```python
from build123d import *

# Parameters (mm, degrees)
CROQUIS1_R              = 100
SALIENTE_EXTRUIR1_DEPTH = 3
CROQUIS3_R              = 110
CORTAR_EXTRUIR1_DEPTH   = 3
REDONDEO1_R             = 10
CROQUIS4_R              = 1.5
CORTAR_EXTRUIR2_DEPTH   = 142.453172607
CROQUIS5_R              = 1.25
CROQUIS5_W              = 4.4
CROQUIS5_H              = 7.75
CROQUIS5_W_2            = 7.75
CROQUIS5_H_2            = 4.4
CORTAR_EXTRUIR3_DEPTH   = 142.453172607
CROQUIS6_R              = 20
CORTAR_EXTRUIR4_DEPTH   = 142.453172607


with BuildPart() as part:
    # Croquis1 → Saliente-Extruir1 (new body)
    with BuildSketch(Plane.XY):
        Circle(CROQUIS1_R)
    extrude(amount=SALIENTE_EXTRUIR1_DEPTH)

    # Croquis3 → Cortar-Extruir1 (cut)
    with BuildSketch(Plane.XY.offset(3)):
        with Locations((190, 0)):
            Circle(CROQUIS3_R)
    extrude(amount=-CORTAR_EXTRUIR1_DEPTH, mode=Mode.SUBTRACT)

    # Redondeo1
    redondeo1_edges = [part.edges().sort_by_distance(p)[0] for p in [
        (89.473684211, -44.659375654, 1.5),
        (89.473684211, 44.659375654, 1.5),
    ]]
    fillet(redondeo1_edges, radius=REDONDEO1_R)

    # Croquis4 → Cortar-Extruir2 (cut, through all)
    with BuildSketch(Plane.XY.offset(3)):
        with Locations((-10.995510447, 37.794857454)):
            Circle(CROQUIS4_R)
        with Locations((-51.936993078, -25.137646071)):
            Circle(CROQUIS4_R)
        with Locations((-25.137646071, -51.936993078)):
            Circle(CROQUIS4_R)
        with Locations((-10.995510447, -37.794857454)):
            Circle(CROQUIS4_R)
        with Locations((-37.794857454, -10.995510447)):
            Circle(CROQUIS4_R)
        with Locations((-37.794857454, 10.995510447)):
            Circle(CROQUIS4_R)
        with Locations((-51.936993078, 25.137646071)):
            Circle(CROQUIS4_R)
        with Locations((-25.137646071, 51.936993078)):
            Circle(CROQUIS4_R)
        with Locations((37.794857454, 10.995510447)):
            Circle(CROQUIS4_R)
        with Locations((10.995510447, 37.794857454)):
            Circle(CROQUIS4_R)
        with Locations((25.137646071, 51.936993078)):
            Circle(CROQUIS4_R)
        with Locations((51.936993078, 25.137646071)):
            Circle(CROQUIS4_R)
        with Locations((10.995510447, -37.794857454)):
            Circle(CROQUIS4_R)
        with Locations((37.794857454, -10.995510447)):
            Circle(CROQUIS4_R)
        with Locations((51.936993078, -25.137646071)):
            Circle(CROQUIS4_R)
        with Locations((25.137646071, -51.936993078)):
            Circle(CROQUIS4_R)
        Polygon((-83.085046789, -58.336309448), (-58.336309448, -83.085046789), (-43.487067043, -68.235804385), (-68.235804385, -43.487067043), align=None)
        Polygon((-58.336309448, 83.085046789), (-43.487067043, 68.235804385), (-68.235804385, 43.487067043), (-83.085046789, 58.336309448), align=None)
        Polygon((83.085046789, 58.336309448), (68.235804385, 43.487067043), (43.487067043, 68.235804385), (58.336309448, 83.085046789), align=None)
        Polygon((58.336309448, -83.085046789), (43.487067043, -68.235804385), (68.235804385, -43.487067043), (83.085046789, -58.336309448), align=None)
    extrude(amount=-CORTAR_EXTRUIR2_DEPTH, mode=Mode.SUBTRACT)

    # Croquis5 → Cortar-Extruir3 (cut, through all)
    with BuildSketch(Plane.XY.offset(3)):
        with Locations((-86, 18.59)):
            Circle(CROQUIS5_R)
        with Locations((-77, 18.59)):
            Circle(CROQUIS5_R)
        with Locations(Location((-77, -18.59, 0), (0, 0, 180))):
            Circle(CROQUIS5_R)
        with Locations(Location((-86, -18.59, 0), (0, 0, 180))):
            Circle(CROQUIS5_R)
        with Locations((18.59, 77)):
            Circle(CROQUIS5_R)
        with Locations((18.59, 86)):
            Circle(CROQUIS5_R)
        with Locations(Location((-18.59, 86, 0), (0, 0, 180))):
            Circle(CROQUIS5_R)
        with Locations(Location((-18.59, 77, 0), (0, 0, 180))):
            Circle(CROQUIS5_R)
        with Locations((62, 18.59)):
            Circle(CROQUIS5_R)
        with Locations((71, 18.59)):
            Circle(CROQUIS5_R)
        with Locations((62, -18.59)):
            Circle(CROQUIS5_R)
        with Locations((71, -18.59)):
            Circle(CROQUIS5_R)
        with Locations((-18.59, -77)):
            Circle(CROQUIS5_R)
        with Locations((-18.59, -86)):
            Circle(CROQUIS5_R)
        with Locations(Location((18.59, -86, 0), (0, 0, 180))):
            Circle(CROQUIS5_R)
        with Locations(Location((18.59, -77, 0), (0, 0, 180))):
            Circle(CROQUIS5_R)
        with Locations((-14.64, 82.125)):
            Rectangle(CROQUIS5_W, CROQUIS5_H)
        with Locations((-80.875, 14.64)):
            Rectangle(CROQUIS5_W_2, CROQUIS5_H_2)
        with Locations((67.125, 14.64)):
            Rectangle(CROQUIS5_W_2, CROQUIS5_H_2)
        with Locations((-14.64, -80.875)):
            Rectangle(CROQUIS5_W, CROQUIS5_H)
    extrude(amount=-CORTAR_EXTRUIR3_DEPTH, mode=Mode.SUBTRACT)

    # Croquis6 → Cortar-Extruir4 (cut, through all)
    with BuildSketch(Plane(origin=(0, 0, 0), x_dir=(-1, 0, 0), z_dir=(0, 0, -1))):
        Circle(CROQUIS6_R)
    extrude(amount=-CORTAR_EXTRUIR4_DEPTH, mode=Mode.SUBTRACT)


solid = part.part
```
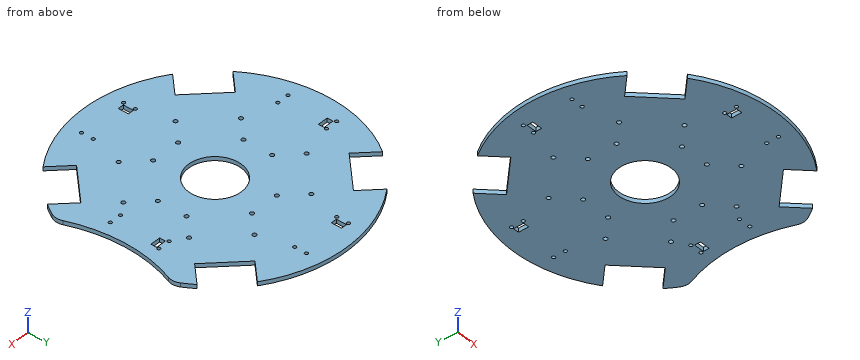
Source: CAD feature listing. Evaluate the final solid. Frame: model axes, mm. Coordinates: 2 decimals unless noted, no trailing zeros. Loops run counter-clockwise (first coordinate to the right, second up) from the corner with the lowest first, then second, coordinate; pieces in that order, holes last. Notation, with made-up numbers: M -34.5,-12.5 L -6.5,-12.5 A18 ccw -6.5,-3.5 Z; hole C 12,14 d7. An arc over 180 degrees is marked long. Use a Markdown table: item, result. Add a question column.
Q1. Section query C-C, the plane z = 0.85. State how many separate pieces and enclosed holes the cut face has, and give its area (3 significant figures).
Q2. Section query D-D, the plane y = 31. Return loops of the section in (x, z).
Q3. Section query A-A, the plane y = 0. Return loops of the section in (x, z), and give its area (3 significant figures).
Q4. First-contact query: pin 1 (2.5 mm diameter, centred on x = -51.94, y = 25.14, fed in from -Z); pin 2 (1 mm diameter, centred on y = 2.5, z = 1, fed in from -X); pin 3 (1.5 mm diameter, centred on y = 15.5, z = 2, fed in from +X); pin 4 (1 mm diameter, centred on x = -51, z = 1.5, fed in from -Y). Flat tips, straight axial feed; report the tip coordinate or a pass-through.
Q5. Material intervals for L1, parallel to X at y = 76.5, z = 1.85; L2, parallel to X at y = 14, z = 0.15; L3, parallel to X at y = 14.5, z = 0.4, sorted ascending.
Q6. Section query B-B, the plane x = 76.5. Return loops of the section in (y, z), and give its area (3 significant figures).
Result:
| question | item | result |
|---|---|---|
| 1 | separate pieces | 1 |
| 1 | enclosed holes | 37 |
| 1 | area | 25,800 mm2 |
| 2 | outline | M -95.07,0 L 84.46,0 L 84.46,3 L -95.07,3 Z |
| 3 | outline | M -100,0 L -20,0 L -20,3 L -100,3 Z; M 20,0 L 80,0 L 80,3 L 20,3 Z |
| 3 | area | 420 mm2 |
| 4 | pin 1 | passes through |
| 4 | pin 2 | stops at x = -99.98 |
| 4 | pin 3 | stops at x = 81.21 |
| 4 | pin 4 | stops at y = -86.31 |
| 5 | L1 | x = -51.75 to -19.74, -17.44 to 17.44, 19.74 to 51.75 |
| 5 | L2 | x = -99.02 to -84.75, -77 to -14.28, 14.28 to 63.25, 71 to 80.89 |
| 5 | L3 | x = -98.94 to -84.75, -77 to -13.77, 13.77 to 63.25, 71 to 80.96 |
| 6 | outline | M -51.75,0 L 51.75,0 L 51.75,3 L -51.75,3 Z |
| 6 | area | 311 mm2 |
